```python
from build123d import *

# Parameters (mm, degrees)
F1_DEPTH = 25
F3_DEPTH = 25


with BuildPart() as f1:
    # F0 (on Front) → F1 (new body, symmetric)
    with BuildSketch(Plane.XZ):
        Polygon((-25, 25), (-25, -25), (-10, -25), (-10, -5), (10, -5), (10, -25), (25, -25), (25, 25), align=None)
    extrude(amount=F1_DEPTH, both=True)

    # F2 (on Right) → F3 (join, symmetric)
    with BuildSketch(Plane.YZ):
        Polygon((25, -25), (25, 25), (-25, 25), (-25, -25), (-10, -25), (-10, -5), (10, -5), (10, -25), align=None)
    extrude(amount=F3_DEPTH, both=True)


solid = f1.part
```
Geometry: final body of the model. Coordinates: model frame, mm. A direction names the side the tool comes from. Coordinates: 2 decimals unless noted, no trailing zeros. Order: outer loops, then holes, each group sorted by start corner. A loop starts at its lowest first (then second) coordinate and runs counter-clockwise, first axis right, second up. Notation, with made-up numbers: (35, 75.25) -> (72, 75.25) arc R14 cw to (72, 99.25) -> close; hole circle Ø7 at (11.5, 87.5). An arc over 180 degrees is marked (long way). Use CSV: the item, a comma, the result in double quotes.
1) Section B-B on z = -19.5. Output: boundary loops of the cut face in (x, y), then the cut area to 3 significant figures.
Findings:
outline,"(-25, -25) -> (25, -25) -> (25, 25) -> (-25, 25) -> close; hole (-10, -10) -> (10, -10) -> (10, 10) -> (-10, 10) -> close"
area,"2,100 mm^2"
2) Line query: line 1 (Y direction, x = 8.5, z = -18.5); line 2 (Z direction, x = -9, y = 1.5). Output: solid intervals per line, ascending.
Findings:
line 1,"y = -25 to -10, 10 to 25"
line 2,"z = -5 to 25"
3) Mould query, pull axis X, two halves, no side actions, for faces 1 (the flat face through (0, 25, 0)), 2 (the flat face through (-25, 0, 0)), 3 (the flat face through (0, -10, -15)). Classes: +X half, -X half, draft (parallel to the pull), parting line (faces both ways), or undercut.
Findings:
face 1,"draft"
face 2,"-X half"
face 3,"undercut"
4) Pin query (flat end, axial travel): pin 1 Ø6 at (x, y) = (1.5, -3.5) entering from -Z. Return the tip coordinate at first contact, or that it passes through.
Findings:
pin 1,"stops at z = -5"
5) Section A-A on x = 6. Output: boundary loops of the cut face in (y, z).
Findings:
outline,"(-25, -25) -> (-10, -25) -> (-10, -5) -> (10, -5) -> (10, -25) -> (25, -25) -> (25, 25) -> (-25, 25) -> close"
6) Access query for faces 4 (the flat face through (0, -25, 0)), 5 (the flat face through (10, 0, -15)). Directions: +Z, -Z, +X, -X, +Y, -Y. A direction counts if a zero-diameter tool reaches every point of the face in a straight line with its end or side. Return the directions, or none.
Findings:
face 4,"+Z, -Z, +X, -X, -Y"
face 5,"-Z"
